```python
from build123d import *

# Parameters (mm, degrees)
F4_R     = 3.175
F5_DEPTH = 76.2


with BuildPart() as f2:
    # F1 (on Top) → F2 (revolve)
    with BuildSketch(Plane.XY):
        with BuildLine():
            Line((0, -19.05), (0, 19.05))
            ThreePointArc((0, 19.05), (-19.05, 0), (0, -19.05))
        make_face()
    revolve(axis=Axis((0, 0, 0), (0, -1, 0)))


with BuildPart() as f5:
    # F4 (on offset) → F5 (new body)
    with BuildSketch(Plane.XZ.offset(-3.175)):
        Circle(F4_R)
    extrude(amount=-F5_DEPTH)


with BuildPart() as f2_1:
    add(f2.part)

    # F6: cut F5
    add(f5.part, mode=Mode.SUBTRACT)


solid = f2_1.part
```
Verification items for the finished model (mm, model axes). Coordinates: 2 decimals unless noted, no trailing zeros. Order: outer loops, then holes, each group sorted by start corner. A loop starts at its lowest first (then second) coordinate and runs counter-clockwise, first axis right, second up. Notation, with made-up numbers: (8.5, 3.5) -> (43.5, 3.5) arc R31 ccw to (43.5, 33.5) -> close; hole circle Ø10 at (6, 87.25). An arc over 180 degrees is marked (long way). Put each result on its own line as item: value. Start each with the question number.
1) Cross-section at A-A (x = 0). Enter the section's corners in (y, z) (3 decimals).
2) Cross-section at B-B (z = 0). Enter the section's corners in (x, y) (3 decimals).
3) Go/stop test with flat-tipped pins: pin 1 (12 mm diameter, centred on y = 12, z = -8, fed in from +X); pin 2 (8 mm diameter, centred on x = 4.5, y = 8.5, fed in from +Z); pin 3 (1.5 mm diameter, centred on x = -14, y = -10, fed in from +Z). Record where each tip stops, or that it passes through.
4) Cross-section at C-C (y = 10). Enter the section's corners in (x, z) (3 decimals).
5) Cross-section at D-D (y = -11). Enter the section's corners in (x, z).
6) Material ranges on L1, parallel to Z at x = 0, y = 6.75 (3 decimals); L2, parallel to Z at x = 0, y = 9 (3 decimals); L3, parallel to X at y = 8, z = 2, recorded low to high.
Geometry check:
1. outline: (3.175, -3.175) -> (3.175, 3.175) -> (18.784, 3.175) arc R19.05 ccw (long way) to (18.784, -3.175) -> close
2. outline: (-3.175, 3.175) -> (-3.175, 18.784) arc R19.05 ccw (long way) to (3.175, 18.784) -> (3.175, 3.175) -> close
3. pin 1: stops at x = 17.09
3. pin 2: stops at z = 18.2
3. pin 3: stops at z = 9.6
4. outline: circle Ø32.429 at (0, 0); hole circle Ø6.35 at (0, 0)
5. outline: circle Ø31.11 at (0, 0)
6. L1: z = -17.814 to -3.175, 3.175 to 17.814
6. L2: z = -16.79 to -3.175, 3.175 to 16.79
6. L3: x = -17.17 to -2.47, 2.47 to 17.17
